Geometry check sheet. Reference: the model listing, model coordinates, mm. Face numbers are marked on the shaded views. A direction names the side the tool comes from. Give positions to 0.01 mm unless a question says otherwise; leave off trailing zeros. Write each loop counter-clockwise with the first axis right and the second up, starting at its lowest first coordinate (ties: lowest second). Pieces come first, ordered by that corner, then holes. Notation, with made-up numbers: M -37.75,-39 L 18.25,-39 A33 cw 18.25,-9 Z; hole C 46,9 d6. An arc over 180 degrees is marked long. One line per item, written item: value. Start each with the question number.
1. Cross-section at C-C on z = 8.25. Record the cut outline in (x, y).
2. Gauge pin test, flat ends, axial feed: pin 1 (1.6 mm diameter, centred on x = 3, z = 7.5, fed in from -Y); pin 2 (1 mm diameter, centred on y = 33, z = 5, fed in from +X); pin 3 (5 mm diameter, centred on y = 60, z = 4, fed in from -X). Record the tip position at first contact, or that the pin passes through.
3. Scan lines: line 1 (Z direction, x = 13.1, y = 60); line 2 (Z direction, x = 0.5, y = 14); line 3 (X direction, y = 9, z = 12.5). Record each from-to range of solid material in increasing order.
4. Cross-section at B-B on y = 60. Record the cut outline in (x, z), then the cut area to 3 significant figures.
5. Tool access check on the marked faces 1, 2 and 3. Record the directions out of +Z, -Z, +X, -X, +Y, -Y that give a thin tool (end or side, any length) a straight path to the whole face; none if there is none.
6. Release check for a two-part mould opening along Z. For the marked faces 4, 5 and 6 record: pulls with the +Z half, pulls with the -Z half, needs draft (parallel to the pull), parting line crosses it, or undercut.
7. Cross-section at D-D on y = 34.5. Record the cut outline in (x, z), then the cut area to 3 significant figures.
8. Cross-section at A-A on z = 12.5. Record the cut outline in (x, y), then the cut area to 3 significant figures.
from build123d import *

# Parameters (mm, degrees)
BOSS_EXTRUDE2_DEPTH = 16.5
SKETCH4_R           = 2.1
CUT_EXTRUDE2_DEPTH  = 16.5
CUT_EXTRUDE3_REACH  = 74.61
SKETCH5_R           = 1.6
FILLET1_R           = 2
FILLET2_R           = 2
CUT_EXTRUDE4_DEPTH  = 2


with BuildPart() as part:
    # Sketch3 → Boss-Extrude2 (new body)
    with BuildSketch(Plane.XY):
        Polygon((0, 0), (0, 20), (10, 50), (10, 70), (14, 70), (14, 49.350889359), (4, 19.350889359), (4, 0), align=None)
    extrude(amount=BOSS_EXTRUDE2_DEPTH)

    # Sketch4 → Cut-Extrude2 (cut)
    with BuildSketch(Plane(origin=(14, 0, 0), x_dir=(0, 0, -1), z_dir=(1, 0, 0))):
        with Locations(Location((-12.5, 60, 0), (0, 0, 90))):
            Circle(SKETCH4_R)
        with Locations(Location((-4, 60, 0), (0, 0, 90))):
            Circle(SKETCH4_R)
    extrude(amount=-CUT_EXTRUDE2_DEPTH, mode=Mode.SUBTRACT)

    # Sketch5 → Cut-Extrude3 (cut, up to next)
    with BuildSketch(Plane(origin=(4, 0, 0), x_dir=(0, 0, -1), z_dir=(1, 0, 0)), mode=Mode.PRIVATE) as cut_extrude3_sk1:
        with Locations(Location((-8.25, 14, 0), (0, 0, 90))):
            Circle(SKETCH5_R)
    cut_extrude3_tool1 = extrude(cut_extrude3_sk1.sketch, amount=-CUT_EXTRUDE3_REACH, mode=Mode.PRIVATE) & part.part
    # Sketch5 → Cut-Extrude3 (cut, up to next)
    with BuildSketch(Plane(origin=(4, 0, 0), x_dir=(0, 0, -1), z_dir=(1, 0, 0)), mode=Mode.PRIVATE) as cut_extrude3_sk2:
        with Locations(Location((-8.25, 6, 0), (0, 0, 90))):
            Circle(SKETCH5_R)
    cut_extrude3_tool2 = extrude(cut_extrude3_sk2.sketch, amount=-CUT_EXTRUDE3_REACH, mode=Mode.PRIVATE) & part.part
    add(cut_extrude3_tool1.solids().sort_by_distance((4, 14, 8.25))[0], mode=Mode.SUBTRACT)
    add(cut_extrude3_tool2.solids().sort_by_distance((4, 6, 8.25))[0], mode=Mode.SUBTRACT)

    # Fillet1
    fillet1_edges = [part.edges().sort_by_distance(p)[0] for p in [
        (14, 70, 8.25),
        (4, 0, 8.25),
    ]]
    fillet(fillet1_edges, radius=FILLET1_R)

    # Fillet2
    # the kernel refuses this fillet: 2 mm, written as the material it takes off along each edge
    with BuildSketch(Plane(origin=(5, 70, 0), x_dir=(0, -1, 0), z_dir=(1, 0, 0))) as fillet2_piece_1:
        with BuildLine():
            CenterArc((FILLET2_R, -FILLET2_R), FILLET2_R, 90, 90)
            Line((0, -FILLET2_R), (0, 0))
            Line((0, 0), (FILLET2_R, 0))
        make_face()
    extrude(amount=12, mode=Mode.SUBTRACT)
    with BuildSketch(Plane(origin=(5, 70, 16.5), x_dir=(0, -1, 0), z_dir=(1, 0, 0))) as fillet2_piece_2:
        with BuildLine():
            CenterArc((FILLET2_R, FILLET2_R), FILLET2_R, 180, 90)
            Line((0, FILLET2_R), (0, 0))
            Line((0, 0), (FILLET2_R, 0))
        make_face()
    extrude(amount=12, mode=Mode.SUBTRACT)

    # Sketch6 → Cut-Extrude4 (cut)
    with BuildSketch(Plane(origin=(4, 0, 0), x_dir=(0, 0, -1), z_dir=(1, 0, 0))):
        Polygon((-5.016838493, 14), (-6.633419246, 16.8), (-9.866580754, 16.8), (-11.483161507, 14), (-9.866580754, 11.2), (-6.633419246, 11.2), align=None)
        Polygon((-6.633419246, 8.8), (-9.866580754, 8.8), (-11.483161507, 6), (-9.866580754, 3.2), (-6.633419246, 3.2), (-5.016838493, 6), align=None)
    extrude(amount=-CUT_EXTRUDE4_DEPTH, mode=Mode.SUBTRACT)


solid = part.part
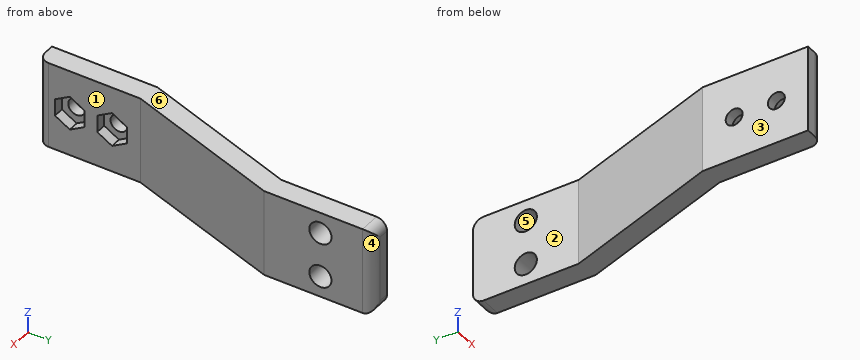
Report:
1. outline: M 0,0 L 2,0 A2 ccw 4,2 L 4,3.2 L 2,3.2 L 2,4.4 L 0,4.4 Z; M 0,7.6 L 2,7.6 L 2,8.8 L 4,8.8 L 4,11.2 L 2,11.2 L 2,12.4 L 0,12.4 Z; M 0,15.6 L 2,15.6 L 2,16.8 L 4,16.8 L 4,19.35 L 14,49.35 L 14,68 A2 ccw 12,70 L 10,70 L 10,50 L 0,20 Z
2. pin 1: stops at y = 0.01
2. pin 2: stops at x = 8.72
2. pin 3: stops at x = 10
3. line 1: z = 0 to 1.9, 6.1 to 10.4, 14.6 to 16.5
3. line 2: z = 0 to 6.65, 9.85 to 16.5
3. line 3: x = 0 to 4
4. outline: M 10,0 L 14,0 L 14,1.9 L 10,1.9 Z; M 10,6.1 L 14,6.1 L 14,10.4 L 10,10.4 Z; M 10,14.6 L 14,14.6 L 14,16.5 L 10,16.5 Z
4. area: 32.4 mm^2
5. face 1: +Z, -Z, +X, -Y
5. face 2: +Z, -Z, -X, +Y
5. face 3: +Z, -Z, -X, +Y, -Y
6. face 4: needs draft
6. face 5: undercut
6. face 6: pulls with the +Z half
7. outline: M 4.83,0 L 9.05,0 L 9.05,16.5 L 4.83,16.5 Z
7. area: 69.6 mm^2
8. outline: M 0,0 L 2,0 A2 ccw 4,2 L 4,19.35 L 14,49.35 L 14,57.9 L 10,57.9 L 10,50 L 0,20 Z; M 10,62.1 L 14,62.1 L 14,68 A2 ccw 12,70 L 10,70 Z
8. area: 268 mm^2
